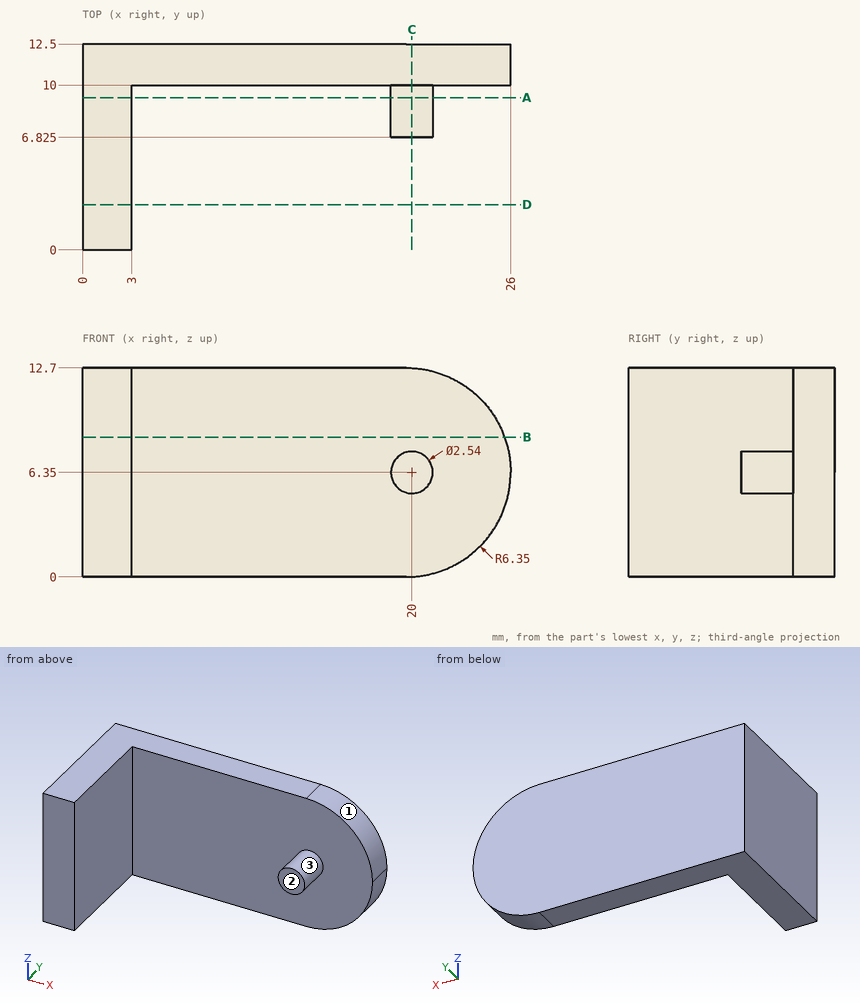
The figure shows three views and two pictorial views of one solid part (mm, origin at its lowest corner). Answer the questions. Give positions to 0.01 mm unless a question says otherwise; leave off trailing zeros. Write each loop counter-clockwise with the first axis right and the second up, starting at its lowest first coordinate (ties: lowest second). Pieces come first, ordered by that corner, then holes. Notation, with made-up numbers: (37, -13) -> (50, -13) arc R35 ccw to (50, 24) -> close; hole circle Ø6 at (-16.75, -12). An arc over 180 degrees is marked (long way). Use one line per item in the form item = value.
1) Section B-B on z = 8.5 is taken. Write down the section's boundary in (x, y).
Result:
outline = (0, 0) -> (3, 0) -> (3, 10) -> (25.62, 10) -> (25.62, 12.5) -> (0, 12.5) -> close
2) Section D-D on y = 2.75 is taken. Write down the section's boundary in (x, z), plus the area to 3 significant figures.
Result:
outline = (0, 0) -> (3, 0) -> (3, 12.7) -> (0, 12.7) -> close
area = 38.1 mm²
3) Section C-C on x = 20 is taken. Write down the section's boundary in (y, z) (3 decimals), plus the area to 3 significant figures.
Result:
outline = (6.825, 5.08) -> (10, 5.08) -> (10, 0.01) -> (12.5, 0.01) -> (12.5, 12.69) -> (10, 12.69) -> (10, 7.62) -> (6.825, 7.62) -> close
area = 39.8 mm²
4) Straight lines are drawn through the part: probe 1 along X at (y, z) = (5.5, 10); probe 2 along Y at (x, z) = (24.5, 3.5); probe 3 along X at (y, z) = (7.25, 7). For each, find the intervals that lie inside material, in ascending order.
Result:
probe_1 = 0 to 3
probe_2 = 10 to 12.5
probe_3 = 0 to 3, 18.91 to 21.09
5) For a pull along X with two mould halves and no side action, classify the marked faces 1, 2 and 3 as +X half, -X half, draft (parallel to the pull), parting line (faces both ways), or undercut.
Result:
face_1 = +X half
face_2 = draft
face_3 = undercut
6) Section A-A on y = 9.25 is taken. Write down the section's boundary in (x, z).
Result:
outline = (0, 0) -> (3, 0) -> (3, 12.7) -> (0, 12.7) -> close; circle Ø2.54 at (20, 6.35)
7) Each of these flat-tipped pins is pushed along its axis until it touches: P1, Ø3, axis at y = 7, z = 2.5, coming from the +X side; P2, Ø2, axis at x = 19.5, z = 6.5, coming from the -Y side (3 decimals); P3, Ø1, axis at x = 22, y = 7, coming from the -Z side; P4, Ø4, axis at x = 11, z = 11, coming from the -Y side. Where does it stop, or does it pass through?
Result:
P1 = 3
P2 = 6.825
P3 = through
P4 = 10
